from build123d import *

# Parameters (mm, degrees)
SALIENTE_EXTRUIR1_DEPTH = 25
VACIADO1_T              = -2
CORTAR_EXTRUIR1_REACH   = 27
CROQUIS3_R              = 3.5
SALIENTE_EXTRUIR2_DEPTH = 25
REDONDEO1_R             = 2
REDONDEO2_R             = 2


with BuildPart() as part:
    # Croquis1 → Saliente-Extruir1 (new body)
    with BuildSketch(Plane(origin=(0, 0, 0), x_dir=(1, 0, 0), z_dir=(0, 1, 0))):
        with BuildLine():
            Line((57.240287673, 0), (120, 0))
            Line((120, 0), (120, 45.324457228))
            Line((120, 45.324457228), (57.240287673, 45.324457228))
            ThreePointArc((57.240287673, 45.324457228), (40.867200252, 48.081235404), (26.299591633, 56.047576896))
            ThreePointArc((26.299591633, 56.047576896), (-42.5, 22.662228614), (26.299591633, -10.723119668))
            ThreePointArc((26.299591633, -10.723119668), (40.867200252, -2.756778176), (57.240287673, 0))
        make_face()
    extrude(amount=SALIENTE_EXTRUIR1_DEPTH)

    # Vaciado1
    vaciado1_openings = [part.faces().sort_by_distance(p)[0] for p in [
        (56.079114696, 0, -22.662228614),
    ]]
    offset(amount=VACIADO1_T, openings=vaciado1_openings, kind=Kind.INTERSECTION)

    # Croquis3 → Cortar-Extruir1 (cut, up to next)
    with BuildSketch(Plane(origin=(0, 25, 0), x_dir=(1, 0, 0), z_dir=(0, 1, 0)), mode=Mode.PRIVATE) as cortar_extruir1_sk1:
        with Locations((0, 54.662228614)):
            Circle(CROQUIS3_R)
    cortar_extruir1_tool1 = extrude(cortar_extruir1_sk1.sketch, amount=-CORTAR_EXTRUIR1_REACH, mode=Mode.PRIVATE) & part.part
    add(cortar_extruir1_tool1.solids().sort_by_distance((0, 25, -54.662229))[0], mode=Mode.SUBTRACT)
    # Croquis3 → Cortar-Extruir1 (cut, up to next)
    with BuildSketch(Plane(origin=(0, 25, 0), x_dir=(1, 0, 0), z_dir=(0, 1, 0)), mode=Mode.PRIVATE) as cortar_extruir1_sk2:
        with Locations((0, -9.337771386)):
            Circle(CROQUIS3_R)
    cortar_extruir1_tool2 = extrude(cortar_extruir1_sk2.sketch, amount=-CORTAR_EXTRUIR1_REACH, mode=Mode.PRIVATE) & part.part
    add(cortar_extruir1_tool2.solids().sort_by_distance((0, 25, 9.337771))[0], mode=Mode.SUBTRACT)

    # Croquis4 → Saliente-Extruir2 (add)
    with BuildSketch(Plane(origin=(0, 25, 0), x_dir=(1, 0, 0), z_dir=(0, 1, 0))):
        Polygon((120, 45.324457228), (120, 50.324457228), (117, 50.324457228), (115, 45.324457228), align=None)
        Polygon((115, 0), (120, 0), (120, -5), (117, -5), align=None)
    extrude(amount=-SALIENTE_EXTRUIR2_DEPTH)

    # Redondeo1
    redondeo1_edges = [part.edges().sort_by_distance(p)[0] for p in [
        (40.867200252, 25, 2.756778176),
        (86.120143836, 25, 0),
        (40.867200252, 25, -48.081235404),
        (86.120143836, 25, -45.324457228),
        (-42.5, 25, -22.662228614),
    ]]
    fillet(redondeo1_edges, radius=REDONDEO1_R)

    # Redondeo2
    redondeo2_edges = [part.edges().sort_by_distance(p)[0] for p in [
        (40.212276755, 23, -46.191506531),
        (-40.5, 23, -22.662228614),
        (40.212276755, 23, 0.867049303),
        (87.620143836, 23, -2),
        (118, 23, -22.662228614),
        (87.620143836, 23, -43.324457228),
    ]]
    fillet(redondeo2_edges, radius=REDONDEO2_R)


solid = part.part
The listing builds one solid part. Answer for the finished solid, in the listing's coordinates (mm). A direction names the side the tool comes from. Give positions to 0.01 mm unless a question says otherwise; leave off trailing zeros. Loops run counter-clockwise (first coordinate to the right, second up) from the corner with the lowest first, then second, coordinate; pieces in that order, holes last.
Item 1: Each of these flat-tipped pins is pushed along its axis until it touches: pin 1 Ø11 at (x, z) = (0, -54.66) entering from -Y; pin 2 Ø3 at (x, y) = (-21.5, 13.5) entering from +Z; pin 3 Ø2 at (y, z) = (15, -30) entering from -X; pin 4 Ø8 at (x, z) = (0, 9.34) entering from +Y. Where does it stop, or does it pass through?
Derived:
pin 1: stops at y = 23
pin 2: stops at z = 14.84
pin 3: stops at x = -42.02
pin 4: stops at y = 25
Item 2: A cutting plane is placed at A-A (x = 71). Give the vertices of the cut face in (y, z), then the cut area to 3 significant figures.
Derived:
outline: (0, -45.32) - (23, -45.32) arc R2 ccw to (25, -43.32) - (25, -2) arc R2 ccw to (23, 0) - (0, 0) - (0, -2) - (21, -2) arc R2 cw to (23, -4) - (23, -41.32) arc R2 cw to (21, -43.32) - (0, -43.32) - close
area: 183 mm2
Item 3: A cutting plane is placed at B-B (x = 0). Give the number of separate pieces and of enclosed holes in the cut face, then the cut area to 3 significant figures.
Derived:
separate pieces: 3
enclosed holes: 0
area: 234 mm2
Item 4: Determine the mould class of faces 1 (the flat face through (120, 13, -22)), 2 (the cylindrical face through (41.1, 11.3, -48)), 3 (the flat face through (119, 13, 5)) for opening direction X: +X half, -X half, draft (parallel to the pull), parting line (faces both ways), or undercut.
Derived:
face 1: +X half
face 2: undercut
face 3: draft
Item 5: A tool of negligible diameter and unlimited length cuts with its end or side. For faces 4 (the cylindrical face through (40.647, 11.339, 2.834)), 5 (the flat face through (38, 23, -23)), 6 (the flat face through (119, 13, -50.324)), 7 (the cylindrical face through (-0.759, 24.014, 12.755)), from which of +Z, -Z, +X, -X, +Y, -Y can it reach the whole face along a straight path? Write none if from no direction.
Derived:
face 4: +Z, +Y, -Y
face 5: -Y
face 6: -Z, +X, +Y, -Y
face 7: +Y, -Y
Item 6: Find the intervals of material crossed by line 1 along Z through (x, y) = (0, 24.4); line 2 along Z through (x, y) = (75, 19); line 3 along Z through (x, y) = (0, 24.2), in increasing order.
Derived:
line 1: z = -64.59 to -58.16, -51.16 to 5.84, 12.84 to 19.27
line 2: z = -45.32 to -43.32, -2 to 0
line 3: z = -64.76 to -58.16, -51.16 to 5.84, 12.84 to 19.44
